Geometry check sheet. Reference: drawing and pictorial views, mm from the part's lowest x, y, z. A direction names the side the tool comes from. Round coordinates to 2 decimals unless told otherwise and drop trailing zeros. Write each loop counter-clockwise with the first axis right and the second up, starting at its lowest first coordinate (ties: lowest second). Pieces come first, ordered by that corner, then holes. Notation, with made-up numbers: M -13.75,31.25 L -2.75,31.25 A11 cw -2.75,52.25 Z; hole C -3,70.5 d3. An arc over 180 degrees is marked long. Put each result on its own line as item: value. Start each with the question number.
(1) Section check A-A on z = 2.5. Count the separate pieces of the cut face and the enclosed holes in it, then the cut area to 3 significant figures.
(2) Section check C-C on x = 22.75. Record the cut outline in (y, z), then the cut area to 3 significant figures.
(3) Mould release check, pull along X, two halves, no side actions. Record for the marked faces 1, 2, 3 and 4: pulls with the +X half, pulls with the -X half, needs draft (parallel to the pull), parting line crosses it, or undercut.
(4) Tool access check on the marked faces 5 and 6. Record the directions out of +Z, -Z, +X, -X, +Y, -Y that give a thin tool (end or side, any length) a straight path to the whole face; none if there is none.
(5) Gauge pin test, flat ends, axial feed: pin 1 (2 mm diameter, centred on x = 3.5, y = 6.5, fed in from -Z); pin 2 (1 mm diameter, centred on x = 15, y = 5, fed in from -Z); pin 3 (1.5 mm diameter, centred on x = 3, z = 4, fed in from -Y). Record the tip position at first contact, or that the pin passes through.
(6) Material ranges on probe 1 along Z at (x, y) = (6.75, 4.75), recorded low to high.
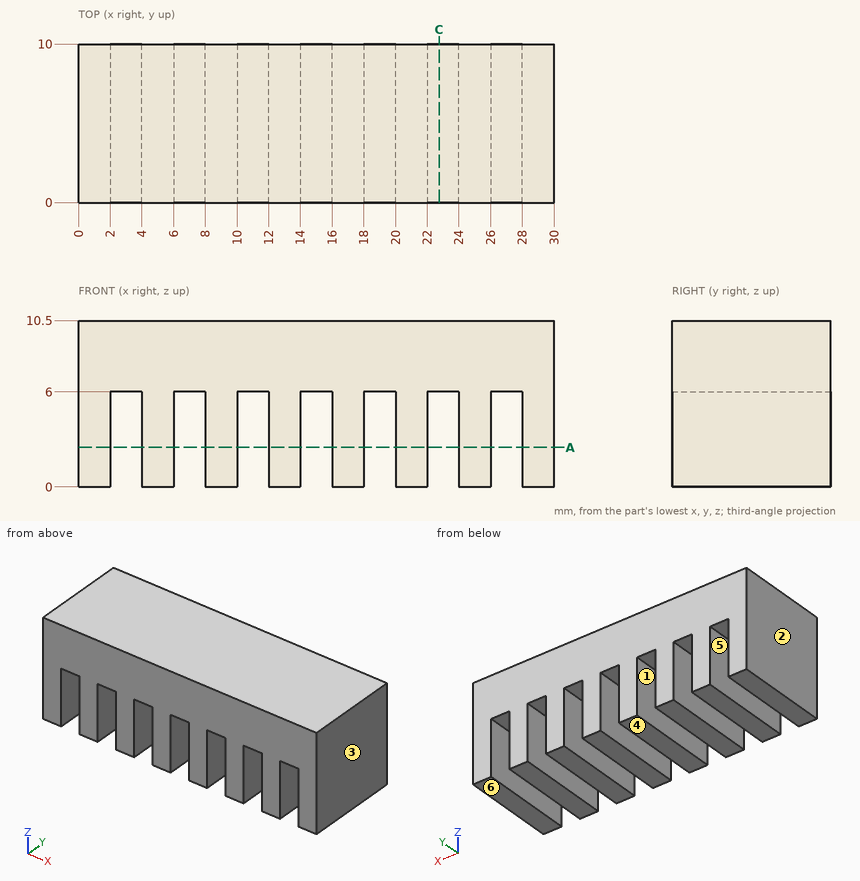
Answers follow:
1. separate pieces: 8
1. enclosed holes: 0
1. area: 160 mm^2
2. outline: M 0,6 L 10,6 L 10,10.5 L 0,10.5 Z
2. area: 45.0 mm^2
3. face 1: undercut
3. face 2: pulls with the -X half
3. face 3: pulls with the +X half
3. face 4: needs draft
4. face 5: -Z, +Y, -Y
4. face 6: -Z, +X, -X, +Y, -Y
5. pin 1: stops at z = 0
5. pin 2: stops at z = 6
5. pin 3: passes through
6. probe 1: z = 6 to 10.5
